```python
from build123d import *

# Parameters (mm, degrees)
EXTRUDE_1_DEPTH     = 45
EXTRUDE_2_DEPTH     = 2
SKETCH_5_W          = 5
SKETCH_5_H          = 5
CUT_EXTRUDE_1_DEPTH = 46


with BuildPart() as part:
    # Эскиз1 → Бобышка-Вытянуть1 (new body)
    with BuildSketch(Plane.XY):
        with BuildLine():
            Line((0, 0), (0, 6))
            ThreePointArc((0, 6), (25, 16.355339059), (50, 6))
            Line((50, 6), (50, 0))
            Line((50, 0), (50, -4))
            Line((50, -4), (42, -4))
            Line((42, -4), (42, -2))
            Line((42, -2), (47.5, -2))
            Line((47.5, -2), (47.5, 0))
            Line((47.5, 0), (47.5, 4.5))
            ThreePointArc((47.5, 4.5), (25, 13.819805153), (2.5, 4.5))
            Line((2.5, 4.5), (2.5, 0))
            Line((2.5, 0), (2.5, -2))
            Line((2.5, -2), (8, -2))
            Line((8, -2), (8, -4))
            Line((8, -4), (0, -4))
            Line((0, -4), (0, 0))
        make_face()
    extrude(amount=EXTRUDE_1_DEPTH)

    # Эскиз3 → Бобышка-Вытянуть2 (add)
    with BuildSketch(Plane.XY.offset(45)):
        with BuildLine():
            Line((0, -4), (50, -4))
            Line((50, -4), (50, 6))
            ThreePointArc((50, 6), (25, 16.355339059), (0, 6))
            Line((0, 6), (0, -4))
        make_face()
    extrude(amount=EXTRUDE_2_DEPTH)

    # Эскиз5 → Вырез-Вытянуть1 (cut)
    with BuildSketch(Plane(origin=(0, 4, 0), x_dir=(1, 0, 0), z_dir=(0, 1, 0))):
        with Locations((15, -6.5)):
            Rectangle(SKETCH_5_W, SKETCH_5_H)
        with Locations((5, -6.5)):
            Rectangle(SKETCH_5_W, SKETCH_5_H)
        with Locations((25, -6.5)):
            Rectangle(SKETCH_5_W, SKETCH_5_H)
        with Locations((35, -6.5)):
            Rectangle(SKETCH_5_W, SKETCH_5_H)
        with Locations((45, -6.5)):
            Rectangle(SKETCH_5_W, SKETCH_5_H)
        with Locations((15, -16.5)):
            Rectangle(SKETCH_5_W, SKETCH_5_H)
        with Locations((5, -16.5)):
            Rectangle(SKETCH_5_W, SKETCH_5_H)
        with Locations((25, -16.5)):
            Rectangle(SKETCH_5_W, SKETCH_5_H)
        with Locations((35, -16.5)):
            Rectangle(SKETCH_5_W, SKETCH_5_H)
        with Locations((45, -16.5)):
            Rectangle(SKETCH_5_W, SKETCH_5_H)
        with Locations((15, -26.5)):
            Rectangle(SKETCH_5_W, SKETCH_5_H)
        with Locations((5, -26.5)):
            Rectangle(SKETCH_5_W, SKETCH_5_H)
        with Locations((25, -26.5)):
            Rectangle(SKETCH_5_W, SKETCH_5_H)
        with Locations((35, -26.5)):
            Rectangle(SKETCH_5_W, SKETCH_5_H)
        with Locations((45, -26.5)):
            Rectangle(SKETCH_5_W, SKETCH_5_H)
        with Locations((15, -36.5)):
            Rectangle(SKETCH_5_W, SKETCH_5_H)
        with Locations((5, -36.5)):
            Rectangle(SKETCH_5_W, SKETCH_5_H)
        with Locations((25, -36.5)):
            Rectangle(SKETCH_5_W, SKETCH_5_H)
        with Locations((35, -36.5)):
            Rectangle(SKETCH_5_W, SKETCH_5_H)
        with Locations((45, -36.5)):
            Rectangle(SKETCH_5_W, SKETCH_5_H)
    extrude(amount=CUT_EXTRUDE_1_DEPTH, mode=Mode.SUBTRACT)


solid = part.part
```
Here's how the part is built. I have some questions about the finished solid (model axes, mm). A direction names the side the tool comes from. Give positions to 0.01 mm unless a question says otherwise; leave off trailing zeros. Write each loop counter-clockwise with the first axis right and the second up, starting at its lowest first coordinate (ties: lowest second). Pieces come first, ordered by that corner, then holes. Notation, with made-up numbers: M 30,-3.5 L 53,-3.5 A6 ccw 53,4.5 Z; hole C 53.25,82 d8. An arc over 180 degrees is marked long. Put each result on its own line as item: value. Start each with the question number.
Item 1: If we section it at D-D, the plane z = 31.5: Write out the boundary of the cut face in (x, y), then the cut area to 3 significant figures.
Item 2: If we section it at A-A, the plane z = 16.5: Write out the boundary of the cut face in (x, y), then the cut area to 3 significant figures.
Item 3: On a 3-axis mill with a long thin cutter (end or side, diameter ignored), from which of +Z, -Z, +X, -X, +Y, -Y can I reach the whole of each face in a straight line? I mean faces 1 (the flat face through (15, 13, 24)), 2 (the flat face through (5, 8, 24)), 3 (the flat face through (42.5, 10, 27)), 4 (the cylindrical face through (25.35, 13.818, 22.185)). Say none if no direction works.
Item 4: Will these pins go through, and if not, where does the flat tip stop? pin 1 (1 mm diameter, centred on y = 11.5, z = 9.5, fed in from -X); pin 2 (3.5 mm diameter, centred on y = 10.5, z = 26, fed in from +X); pin 3 (3 mm diameter, centred on y = 14.5, z = 5.5, fed in from -X); pin 4 (1.3 mm diameter, centred on x = 35, y = 12.5, fed in from -Z).
Item 5: I need wall thicknesses on L1, parallel to Z at x = 15.5, y = 15; L2, parallel to X at y = 1.5, z = 35.5; L3, parallel to Z at x = 4, y = 4. Which ranges of each line are inside material? Lowest first, please. Write a range as from..to.
Item 6: If we section it at B-B, the plane y = 3.25: Write out the boundary of the cut face in (x, z).
Item 7: If we section it at C-C, the plane x = 25: Write out the boundary of the cut face in (y, z).
Item 8: Thinking about a two-plate mould opening in Z: for faces 5 (the flat face through (7.5, 10, 17)), 6 (the flat face through (25, 15, 0)), which applies, +Z half, -Z half, draft (parallel to the pull), parting line (faces both ways), or undercut?
Values:
1. outline: M 0,-4 L 8,-4 L 8,-2 L 2.5,-2 L 2.5,4.5 A31.82 cw 47.5,4.5 L 47.5,-2 L 42,-2 L 42,-4 L 50,-4 L 50,6 A35.36 ccw 0,6 Z
1. area: 207 mm²
2. outline: M 0,-4 L 8,-4 L 8,-2 L 2.5,-2 L 2.5,8.27 A35.36 ccw 0,6 Z; M 7.5,8.58 A31.82 cw 12.5,11.26 L 12.5,14.07 A35.36 ccw 7.5,11.72 Z; M 17.5,12.92 A31.82 cw 22.5,13.72 L 22.5,16.27 A35.36 ccw 17.5,15.55 Z; M 27.5,13.72 A31.82 cw 32.5,12.92 L 32.5,15.55 A35.36 ccw 27.5,16.27 Z; M 37.5,11.26 A31.82 cw 42.5,8.58 L 42.5,11.72 A35.36 ccw 37.5,14.07 Z; M 42,-4 L 50,-4 L 50,6 A35.36 ccw 47.5,8.27 L 47.5,-2 L 42,-2 Z
2. area: 133 mm²
3. face 1: +Y, -Y
3. face 2: +Y
3. face 3: +X, +Y
3. face 4: -Z
4. pin 1: x = 6.29
4. pin 2: x = 42.5
4. pin 3: x = 9.97
4. pin 4: z = 0
5. L1: 0..4, 9..14, 19..24, 29..34, 39..47
5. L2: 0..2.5, 47.5..50
5. L3: 45..47
6. outline: M 0,0 L 2.5,0 L 2.5,45 L 47.5,45 L 47.5,0 L 50,0 L 50,47 L 0,47 Z
7. outline: M -4,45 L 13.82,45 L 13.82,39 L 16.36,39 L 16.36,47 L -4,47 Z; M 13.82,0 L 16.36,0 L 16.36,4 L 13.82,4 Z; M 13.82,9 L 16.36,9 L 16.36,14 L 13.82,14 Z; M 13.82,19 L 16.36,19 L 16.36,24 L 13.82,24 Z; M 13.82,29 L 16.36,29 L 16.36,34 L 13.82,34 Z
8. face 5: undercut
8. face 6: -Z half
